Answer from the drawing. Dimensions are ordinates in mm from the lowest x, y and z of the part. Coordinates: 2 decimals unless noted, no trailing zeros.
(1) Given pin 1 (12 mm diameter, centred on y = 22.5, z = 12.5, fed in from +X); pin 2 (2 mm diameter, centred on x = 21.5, y = 14.5, fed in from -Z); pin 3 (4 mm diameter, centred on x = 9, z = 11.5, fed in from -Y) (1 decimal), each flat-ended and moving along its own axis, determine where each tip first touches the part or whether it passes through.
(2) Straight lines are drawn through the part: line 1 along X through (y, z) = (18, 2.5) (1 decimal); line 2 along X through (y, z) = (11, 15) (1 decimal); line 3 along Z through (x, y) = (14, 13). For each, find the intervals that lie inside material, in ascending order.
(3) Determine the mould class of the marked faces 1 and 2 for opening direction X: pulls with the +X half, pulls with the -X half, needs draft (parallel to the pull), parting line crosses it, or undercut.
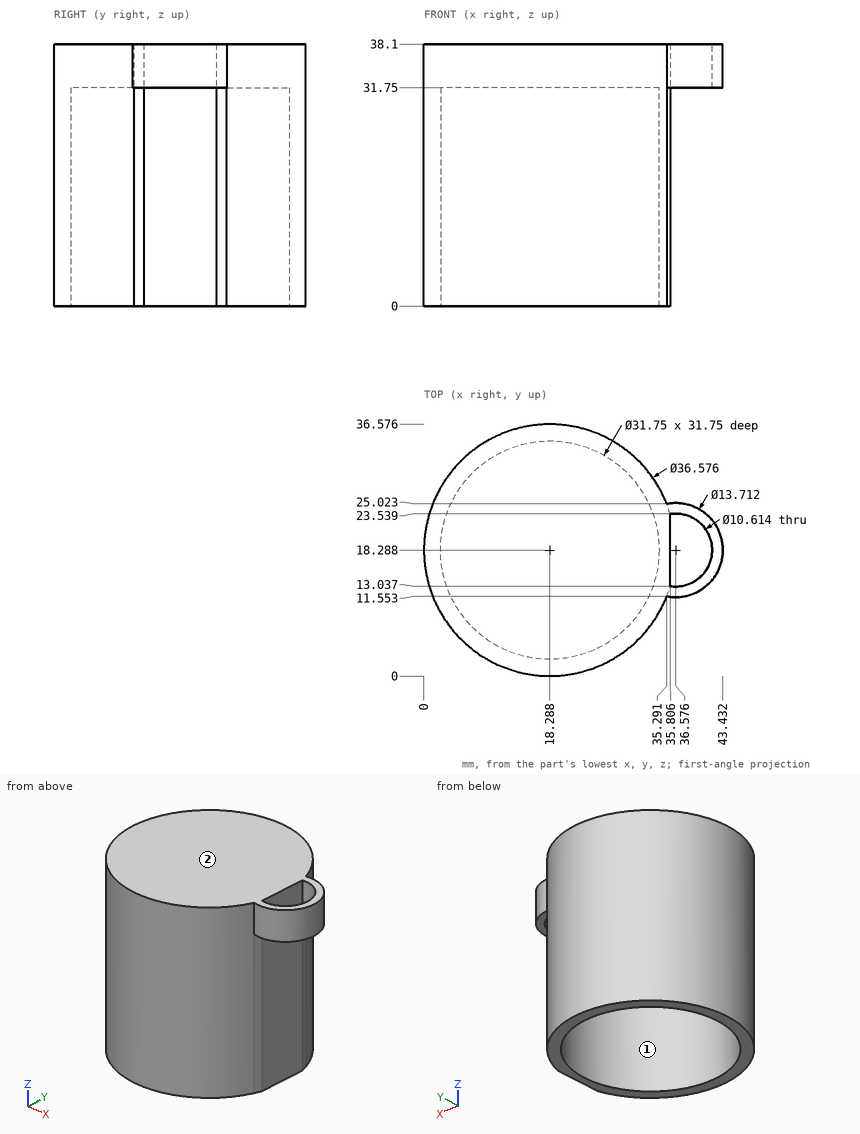
Computed:
1. pin 1: stops at x = 35.81
1. pin 2: stops at z = 31.75
1. pin 3: stops at y = 1.5
2. line 1: x = 0 to 2.4, 34.2 to 35.8
2. line 2: x = 1.5 to 4.2, 32.4 to 35.1
2. line 3: z = 31.75 to 38.1
3. face 1: undercut
3. face 2: needs draft
